Here's how the part is built. I have some questions about the finished solid (model axes, mm). Face numbers are marked on the shaded views. A direction names the side the tool comes from. Round coordinates to 2 decimals unless told otherwise and drop trailing zeros. Order: outer loops, then holes, each group sorted by start corner. A loop starts at its lowest first (then second) coordinate and runs counter-clockwise, first axis right, second up. Notation, with made-up numbers: (38.5, -34) -> (44.5, -34) arc R21 cw to (44.5, -10) -> close; hole circle Ø1 at (65.5, 54). An arc over 180 degrees is marked (long way). Answer in a Markdown table with one row per item.
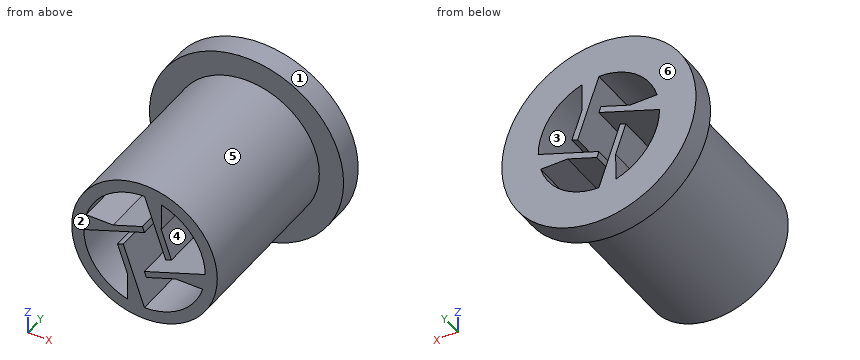
```python
from build123d import *

# Parameters (mm, degrees)
F0_R     = 16
F0_R_2   = 12
F1_DEPTH = 4
F2_DEPTH = 32


with BuildPart() as f1:
    # F0 (on Front) → F1 (new body)
    with BuildSketch(Plane.XZ):
        Circle(F0_R)
        Circle(F0_R_2, mode=Mode.SUBTRACT)
        Circle(F0_R_2)
        with BuildLine():
            ThreePointArc((2.81716, 9.594978), (8.005361, 5.992846), (10, 0))
            ThreePointArc((10, 0), (9.985368, -0.540767), (9.941514, -1.079951))
            ThreePointArc((9.941514, -1.079951), (9.806789, -1.956244), (9.594978, -2.81716))
            ThreePointArc((9.594978, -2.81716), (5.992846, -8.005361), (0, -10))
            ThreePointArc((0, -10), (-0.540767, -9.985368), (-1.079951, -9.941514))
            ThreePointArc((-1.079951, -9.941514), (-1.956244, -9.806789), (-2.81716, -9.594978))
            ThreePointArc((-2.81716, -9.594978), (-8.005361, -5.992846), (-10, 0))
            ThreePointArc((-10, 0), (-9.985368, 0.540767), (-9.941514, 1.079951))
            ThreePointArc((-9.941514, 1.079951), (-9.806789, 1.956244), (-9.594978, 2.81716))
            ThreePointArc((-9.594978, 2.81716), (-5.992846, 8.005361), (0, 10))
            ThreePointArc((0, 10), (0.540767, 9.985368), (1.079951, 9.941514))
            ThreePointArc((1.079951, 9.941514), (1.956244, 9.806789), (2.81716, 9.594978))
        make_face(mode=Mode.SUBTRACT)
    extrude(amount=F1_DEPTH)

    # F0 (on Front) → F2 (join)
    with BuildSketch(Plane.XZ):
        Circle(F0_R_2)
        with BuildLine():
            ThreePointArc((2.81716, 9.594978), (8.005361, 5.992846), (10, 0))
            ThreePointArc((10, 0), (9.985368, -0.540767), (9.941514, -1.079951))
            ThreePointArc((9.941514, -1.079951), (9.806789, -1.956244), (9.594978, -2.81716))
            ThreePointArc((9.594978, -2.81716), (5.992846, -8.005361), (0, -10))
            ThreePointArc((0, -10), (-0.540767, -9.985368), (-1.079951, -9.941514))
            ThreePointArc((-1.079951, -9.941514), (-1.956244, -9.806789), (-2.81716, -9.594978))
            ThreePointArc((-2.81716, -9.594978), (-8.005361, -5.992846), (-10, 0))
            ThreePointArc((-10, 0), (-9.985368, 0.540767), (-9.941514, 1.079951))
            ThreePointArc((-9.941514, 1.079951), (-9.806789, 1.956244), (-9.594978, 2.81716))
            ThreePointArc((-9.594978, 2.81716), (-5.992846, 8.005361), (0, 10))
            ThreePointArc((0, 10), (0.540767, 9.985368), (1.079951, 9.941514))
            ThreePointArc((1.079951, 9.941514), (1.956244, 9.806789), (2.81716, 9.594978))
        make_face(mode=Mode.SUBTRACT)
        with BuildLine():
            ThreePointArc((-1.079951, -9.941514), (-0.540767, -9.985368), (0, -10))
            Line((0, -10), (-3.5, 0))
            Line((-3.5, 0), (-4.443858, -0.33035))
            Line((-4.443858, -0.33035), (-2.761905, -5.135932))
            Line((-2.761905, -5.135932), (-1.079951, -9.941514))
        make_face()
        with BuildLine():
            ThreePointArc((-2.81716, -9.594978), (-1.956244, -9.806789), (-1.079951, -9.941514))
            Line((-1.079951, -9.941514), (-2.761905, -5.135932))
            Line((-2.761905, -5.135932), (-2.81716, -9.594978))
        make_face()
        with BuildLine():
            ThreePointArc((9.941514, -1.079951), (9.985368, -0.540767), (10, 0))
            Line((10, 0), (0, -3.5))
            Line((0, -3.5), (0.33035, -4.443858))
            Line((0.33035, -4.443858), (5.135932, -2.761905))
            Line((5.135932, -2.761905), (9.941514, -1.079951))
        make_face()
        with BuildLine():
            ThreePointArc((9.594978, -2.81716), (9.806789, -1.956244), (9.941514, -1.079951))
            Line((9.941514, -1.079951), (5.135932, -2.761905))
            Line((5.135932, -2.761905), (9.594978, -2.81716))
        make_face()
        with BuildLine():
            Line((2.761905, 5.135932), (1.079951, 9.941514))
            ThreePointArc((1.079951, 9.941514), (0.540767, 9.985368), (0, 10))
            Line((0, 10), (3.5, 0))
            Line((3.5, 0), (4.443858, 0.33035))
            Line((4.443858, 0.33035), (2.761905, 5.135932))
        make_face()
        with BuildLine():
            Line((2.761905, 5.135932), (2.81716, 9.594978))
            ThreePointArc((2.81716, 9.594978), (1.956244, 9.806789), (1.079951, 9.941514))
            Line((1.079951, 9.941514), (2.761905, 5.135932))
        make_face()
        with BuildLine():
            Line((-5.135932, 2.761905), (-9.594978, 2.81716))
            ThreePointArc((-9.594978, 2.81716), (-9.806789, 1.956244), (-9.941514, 1.079951))
            Line((-9.941514, 1.079951), (-5.135932, 2.761905))
        make_face()
        with BuildLine():
            Line((-5.135932, 2.761905), (-9.941514, 1.079951))
            ThreePointArc((-9.941514, 1.079951), (-9.985368, 0.540767), (-10, 0))
            Line((-10, 0), (0, 3.5))
            Line((0, 3.5), (-0.33035, 4.443858))
            Line((-0.33035, 4.443858), (-5.135932, 2.761905))
        make_face()
    extrude(amount=F2_DEPTH)


solid = f1.part
```
1. Please list where these lines run through material, in increasing order: line 1 along X through (y, z) = (-9.5, 7.5) (1 decimal); line 2 along Z through (x, y) = (8, -27); line 3 along X through (y, z) = (-5, -7.5) (1 decimal).
Numbers:
| item | result |
|---|---|
| line 1 | x = -9.4 to -6.6, 0.9 to 2.8, 6.6 to 9.4 |
| line 2 | z = -8.94 to -6, -2.8 to -0.7, 6 to 8.94 |
| line 3 | x = -9.4 to -6.6, -2.8 to -0.9, 6.6 to 9.4 |
2. For the marked faces 4, 5 and 6, which set-ups out of +Z, -Z, +X, -X, +Y, -Y let a thin tool reach every point of the face, with its end or its side?
Numbers:
| item | result |
|---|---|
| face 4 | +Y, -Y |
| face 5 | -Y |
| face 6 | +Z, -Z, +X, -X, +Y |
3. Suppose I cut it at D-D on y = -3. Write out the boundary of the cut face in (x, z).
Numbers:
| item | result |
|---|---|
| outline | circle Ø32 at (0, 0); hole (-10, 0) arc R10 ccw to (-2.82, -9.59) -> (-2.76, -5.14) -> (-4.44, -0.33) -> (-3.5, 0) -> (0, -10) arc R10 ccw to (9.59, -2.82) -> (5.14, -2.76) -> (0.33, -4.44) -> (0, -3.5) -> (10, 0) arc R10 ccw to (2.82, 9.59) -> (2.76, 5.14) -> (4.44, 0.33) -> (3.5, 0) -> (0, 10) arc R10 ccw to (-9.59, 2.82) -> (-5.14, 2.76) -> (-0.33, 4.44) -> (0, 3.5) -> close |
4. Suppose I cut it at B-B on x = 7.5. Write out the boundary of the cut face in (y, z) (1 decimal), then the cut area to 3 significant figures.
Numbers:
| item | result |
|---|---|
| outline | (-32, -9.4) -> (-4, -9.4) -> (-4, -14.1) -> (0, -14.1) -> (0, -6.6) -> (-32, -6.6) -> close; (-32, -2.8) -> (0, -2.8) -> (0, -0.9) -> (-32, -0.9) -> close; (-32, 6.6) -> (0, 6.6) -> (0, 14.1) -> (-4, 14.1) -> (-4, 9.4) -> (-32, 9.4) -> close |
| area | 276 mm2 |
5. We'd pull the mould along Z, two halves only. Please class the marked faces 1, 2 and 3: released by +Z, released by -Z, zero draft, split by the parting line, or undercut.
Numbers:
| item | result |
|---|---|
| face 1 | split by the parting line |
| face 2 | zero draft |
| face 3 | undercut |
6. Suppose I cut it at C-C on z = -2. Write out the boundary of the cut face in (x, y), then the cut area to 3 significant figures.
Numbers:
| item | result |
|---|---|
| outline | (-15.87, -4) -> (-11.83, -4) -> (-11.83, -32) -> (-9.8, -32) -> (-9.8, 0) -> (-15.87, 0) -> close; (-3.86, -32) -> (-2.8, -32) -> (-2.8, 0) -> (-3.86, 0) -> close; (4.29, -32) -> (11.83, -32) -> (11.83, -4) -> (15.87, -4) -> (15.87, 0) -> (4.29, 0) -> close |
| area | 373 mm2 |
7. For pin 1 Ø4 at (y, z) = (-23, -2) entering from -X; pin 2 Ø8 at (x, y) = (1.5, -16.5) entering from +Z; pin 3 Ø1 at (x, y) = (-6.5, -22.5) entering from -Z; pin 4 Ø3 at (x, z) = (-8, 6.5) entering from +Y, each with a flat end and sliding along its axis, tell me the tip position at first contact or that it passes through.
Numbers:
| item | result |
|---|---|
| pin 1 | stops at x = -12 |
| pin 2 | stops at z = 12 |
| pin 3 | stops at z = -10.39 |
| pin 4 | stops at y = 0 |
8. Suppose I cut it at A-A on y = -30. Write out the boundary of the cut face in (x, z), then the cut area to 3 significant figures.
Numbers:
| item | result |
|---|---|
| outline | circle Ø24 at (0, 0); hole (-10, 0) arc R10 ccw to (-2.82, -9.59) -> (-2.76, -5.14) -> (-4.44, -0.33) -> (-3.5, 0) -> (0, -10) arc R10 ccw to (9.59, -2.82) -> (5.14, -2.76) -> (0.33, -4.44) -> (0, -3.5) -> (10, 0) arc R10 ccw to (2.82, 9.59) -> (2.76, 5.14) -> (4.44, 0.33) -> (3.5, 0) -> (0, 10) arc R10 ccw to (-9.59, 2.82) -> (-5.14, 2.76) -> (-0.33, 4.44) -> (0, 3.5) -> close |
| area | 196 mm2 |
